Autodesk Inventor part; units mm, degrees
ref_plane "Start Plane" through (0, 0, 18.4542) normal (0, 0, 1) x (1, 0, 0)
ref_plane "End Plane" through (0, 0, 818.5838) normal (0, 0, 1) x (1, 0, 0)
ref_plane "Work Plane4" through (-691.072, 9, 623.4136) normal (-0.2664258, 0, 0.9638554) x (0.9638554, 0, 0.2664258)
ref_plane "Start Plane" through (0, 0, 18.4542) normal (0, 0, 1) x (1, 0, 0)
ref_plane "End Plane" through (0, 0, 818.5838) normal (0, 0, 1) x (1, 0, 0)
sketch "Sketch" plane through (0, 0, 0) normal (0, 0, 1) x (1, 0, 0)
  line L0 (-15, -9) -> (-15, 9)
  line L1 (-9, 15) -> (9, 15)
  line L2 (15, 9) -> (15, -9)
  line L3 (9, -15) -> (-9, -15)
  arc A0 (-15, -9) -> (-9, -15) centre (-9, -9) ccw
  arc A1 (-9, 15) -> (-15, 9) centre (-9, 9) ccw
  arc A2 (15, 9) -> (9, 15) centre (9, 9) ccw
  arc A3 (9, -15) -> (15, -9) centre (9, -9) ccw
  arc A4 (-9, 12) -> (-12, 9) centre (-9, 9) ccw
  line L4 (-9, 12) -> (9, 12)
  arc A5 (12, 9) -> (9, 12) centre (9, 9) ccw
  line L5 (12, 9) -> (12, -9)
  arc A6 (9, -12) -> (12, -9) centre (9, -9) ccw
  line L6 (9, -12) -> (-9, -12)
  arc A7 (-12, -9) -> (-9, -12) centre (-9, -9) ccw
  line L7 (-12, -9) -> (-12, 9)
  line L8 (0, 22.7397) -> (0, -22.7397) construction
  line L9 (-22.7397, 0) -> (22.7397, 0) construction
  dimension "d7" = 6
  dimension "d10" = 30
  dimension "d11" = 30
  dimension "d12" = 3
  dimension "d15" = 15
  dimension "d16" = 15
extrude "Body" add sketch "Sketch" along normal up to surface (800.1295 mm away) from surface at 18.4542
sketch "Sketch3" plane through (0, 0, 0) normal (0, 0, 1) x (1, 0, 0)
  line L0 (0, 0) -> (10, 0)
ref_plane "Work Plane3" through (0, 0, 0) normal (0, -1, 0) x (1, 0, 0)
ref_plane "Work Plane4" through (-691.072, 9, 623.4136) normal (-0.2664258, 0, 0.9638554) x (0.9638554, 0, 0.2664258)
split "Split1" plane through (-691.072, 9, 623.4136) removes the side toward (-0.2664258, 0, 0.9638554)
ref_plane "Work Plane5" through (-198.6828, -9, 775.0807) normal (-0.9638554, 0, -0.2664258) x (-0.2664258, 0, 0.9638554)
split "Split2" plane through (-198.6828, -9, 775.0807) removes the side toward (-0.9638554, 0, -0.2664258)
ref_plane "Work Plane6" through (-3.9964, -9, 14.4578) normal (0.2664258, 0, -0.9638554) x (-0.9638554, 0, -0.2664258)
split "Split3" plane through (-3.9964, -9, 14.4578) removes the side toward (0.2664258, 0, -0.9638554)
sketch "Sketch4" plane through (0, 0, 0) normal (0, -1, 0) x (1, 0, 0)
  line L0 (-2, 18.4542) -> (12, 18.4542)
  line L1 (-2, 818.5838) -> (12, 818.5838)
  dimension "d18" = 800.1295
equation "\"d7\" = G_IR"
equation "\"d10\" = G_H"
equation "\"d11\" = G_W"
equation "\"d12\" = G_T"
equation "\"d15\" = 0.5 * d10"
equation "\"d16\" = 0.5 * d11"
equation "\"d3\" = G_L"
equation "\"G_W\" = 30"
equation "\"G_H\" = 30"
equation "\"G_T\" = 3"
equation "\"G_IR\" = 6"
equation "\"G_L\" = d18"
equation "\"G_OFFSET_START\" = -18.45422"
equation "\"G_OFFSET_END\" = -11.41625"
equation "\"d13\" = -G_OFFSET_START"
equation "\"d14\" = G_OFFSET_END + B_L"
properties part number "DIN EN 10219-2 - 30 x 30 x 3  - 800.13" material "Steel, Mild"
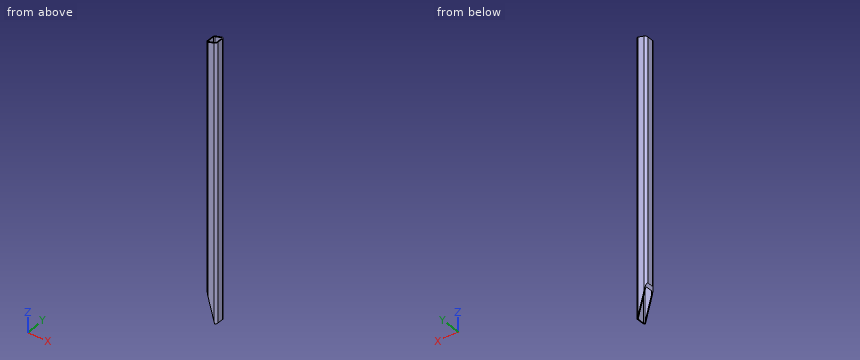
Could you check a few things on this model? Use its own coordinates, in mm. Give positions to 0.01 mm unless a question says otherwise; leave off trailing zeros. Order: outer loops, then holes, each group sorted by start corner. A loop starts at its lowest first (then second) coordinate and runs counter-clockwise, first axis right, second up. Notation, with made-up numbers: (62.25, 80.25) -> (90.25, 80.25) arc R23 cw to (90.25, 109.25) -> close; hole circle Ø8 at (-30, 87.5). An arc over 180 degrees is marked (long way). Answer in a Markdown table with one row per item. Add a question column.
Item 1: Imagine slicing it at C-C (z = 709). List the corners of the cut face in (x, y) for me.
Item 2: Imagine slicing it at B-B (x = 2.5). List the corners of the cut face in (y, z) for me.
Item 3: Imagine slicing it at A-A (y = -1.75). List the corners of the cut face in (x, z) for me, and give its area (3 significant figures).
Item 4: Please list where these lines run through material, in increasing order: probe 1 along Y at (x, z) = (-5.5, 696); probe 2 along X at (y, z) = (9.5, 193); probe 3 along Y at (x, z) = (-10.5, 517.5).
Item 5: I'm going to push flat-ended pins straight in: P1, Ø8, axis at x = -11.5, y = 1.5, coming from the +Z side; P2, Ø1, axis at x = 10.5, z = 141.5, coming from the +Y side; P3, Ø10, axis at x = 9, y = 3.5, coming from the -Z side. Where does each tip first touch, or does it pass through?
Result:
| question | item | result |
|---|---|---|
| 1 | outline | (-15, -9) arc R6 ccw to (-9, -15) -> (9, -15) arc R6 ccw to (15, -9) -> (15, 9) arc R6 ccw to (9, 15) -> (-9, 15) arc R6 ccw to (-15, 9) -> close; hole (-12, -9) arc R3 ccw to (-9, -12) -> (9, -12) arc R3 ccw to (12, -9) -> (12, 9) arc R3 ccw to (9, 12) -> (-9, 12) arc R3 ccw to (-12, 9) -> close |
| 2 | outline | (-15, 47.26) -> (-12, 47.26) -> (-12, 815.13) -> (-15, 815.13) -> close; (12, 47.26) -> (15, 47.26) -> (15, 815.13) -> (12, 815.13) -> close |
| 3 | outline | (-15, 110.57) -> (-12, 99.71) -> (-12, 811.12) -> (-15, 810.29) -> close; (12, 18.88) -> (15, 19.71) -> (15, 818.58) -> (12, 817.75) -> close |
| 3 | area | 4,510 mm2 |
| 4 | probe 1 | -15 to -12, 12 to 15 |
| 4 | probe 2 | -14.98 to -11.96, 11.96 to 14.98 |
| 4 | probe 3 | -14.81 to -11.6, 11.6 to 14.81 |
| 5 | P1 | z = 811.12 |
| 5 | P2 | y = 14.92 |
| 5 | P3 | z = 18.88 |
